Build history of the part. All positions in model axes, mm. Coordinates: 2 decimals unless noted, no trailing zeros. Loops run counter-clockwise (first coordinate to the right, second up) from the corner with the lowest first, then second, coordinate; pieces in that order, holes last.
(1) Two-plate mould, pull along X, no slides. Class faces 1 (the face through (0, 0, 3)), 2 (the face through (-2.17, -9.76, 1.97)), 3 (the face through (0, 0, 0)): pulls with the +X half, pulls with the -X half, needs draft (parallel to the pull), parting line crosses it, or undercut.
(2) Wall check: L1, parallel to Y at x = 0, z = 3.4; L2, parallel to X at y = -6, z = 1. Give the ranges that are in metal, low to high.
(3) Flat gauge pins, fed straight in: P1, Ø2, axis at y = -5, z = 1.5, coming from the +X side; P2, Ø1.5, axis at y = -5.5, z = 2.5, coming from the +X side. Where does each tip first touch, or does it go through?
(4) Slice it at B-B (z = 3.6). Give the cut face in (x, y), and give its area (3 significant figures).
from build123d import *

# Parameters (mm, degrees)
F0_R     = 10
F1_DEPTH = 5
F2_R     = 8
F3_DEPTH = 2
F4_R     = 0.99999


# Not quite as in the source:
# - a fillet or chamfer is up to 0.001 mm smaller than in the source, because OpenCascade refuses the exact size


with BuildPart() as f1:
    # F0 (on Top) → F1 (new body)
    with BuildSketch(Plane.XY):
        Circle(F0_R)
    extrude(amount=F1_DEPTH)

    # F2 (on face) → F3 (cut)
    with BuildSketch(Plane.XY.offset(5)):
        Circle(F2_R)
    extrude(amount=-F3_DEPTH, mode=Mode.SUBTRACT)

    # F4 (radius 1 in the source; OpenCascade refuses exactly that, so slightly less here)
    f4_edges = [f1.edges().sort_by_distance(p)[0] for p in [
        (-10, 0, 5),
        (-8, 0, 5),
    ]]
    fillet(f4_edges, radius=F4_R)


solid = f1.part
Response values:
1. face 1: undercut
1. face 2: parting line crosses it
1. face 3: needs draft
2. L1: y = -10 to -8, 8 to 10
2. L2: x = -8 to 8
3. P1: stops at x = 9.17
3. P2: stops at x = 8.8
4. outline: circle Ø20 at (0, 0); hole circle Ø16 at (0, 0)
4. area: 113 mm2
